Design review of the part built by this model. Coordinates are the model's own, in mm. Face numbers are marked on the shaded views. Coordinates: 2 decimals unless noted, no trailing zeros. Loops run counter-clockwise (first coordinate to the right, second up) from the corner with the lowest first, then second, coordinate; pieces in that order, holes last. Notation, with made-up numbers: (22.25, 16) -> (28.25, 16) arc R33 ccw to (28.25, 45) -> close; hole circle Ø5 at (44.5, 47.5). An arc over 180 degrees is marked (long way). Answer as a JSON object with one key per item and string values.
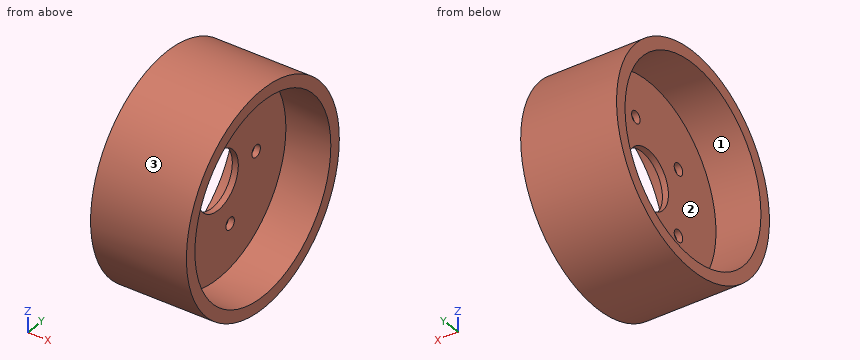
```python
from build123d import *

# Parameters (mm, degrees)
SKETCH1_W                  = 6.35
SKETCH1_H                  = 101.6
SKETCH2_R                  = 30.48
CUT_EXTRUDE2_DEPTH         = 171.417958634
F_1_2_0_5_DIAMETER_HOLE2_D = 12.7


with BuildPart() as part:
    # Sketch1 → Revolve1 (revolve)
    with BuildSketch(Plane.XY):
        with Locations((3.175, 50.8)):
            Rectangle(SKETCH1_W, SKETCH1_H)
        Polygon((-47.625, 101.6), (0, 101.6), (6.35, 101.6), (53.975, 101.6), (53.975, 114.3), (-47.625, 114.3), align=None)
    revolve(axis=Axis((6.35, 0, 0), (-1, 0, 0)))

    # Sketch2 → Cut-Extrude2 (cut, through all)
    with BuildSketch(Plane(origin=(6.35, 0, 0), x_dir=(0, 0, -1), z_dir=(1, 0, 0))):
        with Locations(Location((0, 0, 0), (0, 0, 90))):
            Circle(SKETCH2_R)
    extrude(amount=-CUT_EXTRUDE2_DEPTH, mode=Mode.SUBTRACT)

    # 1/2 (0.5) Diameter Hole2 (through all)
    with Locations(Plane(origin=(6.35, 0, 0), x_dir=(0, 0, -1), z_dir=(1, 0, 0))):
        with Locations((-54.155626078, 18.25625), (0, 57.15), (54.155626078, 18.25625), (34.599427772, -45.486284722), (-34.599427772, -45.486284722)):
            Hole(F_1_2_0_5_DIAMETER_HOLE2_D / 2)


solid = part.part
```
1) Clearance check with flat-ended pins moving along their axes: pin 1 Ø10 at (x, z) = (37, 73) entering from -Y; pin 2 Ø3 at (x, y) = (-10, 56.5) entering from -Z; pin 3 Ø8 at (x, z) = (25.5, -55.5) entering from -Y. State where each tip first meets the part, or that it passes through.
Completed:
{"pin 1": "y = -91.87", "pin 2": "z = -100.2", "pin 3": "y = -102.04"}
2) The part is to be moulded in two halves that separate along Z. For the marked faces 1, 2 and 3, say which applies: pulls with the +Z half, pulls with the -Z half, needs draft (parallel to the pull), parting line crosses it, or undercut.
Completed:
{"face 1": "undercut", "face 2": "undercut", "face 3": "parting line crosses it"}
3) Add section A-A, the plane z = 0. Give the boundary of the cut face in (x, y) (3 decimals), and give its area (3 significant figures).
Completed:
{"outline": "(-47.625, -114.3) -> (53.975, -114.3) -> (53.975, -101.6) -> (6.35, -101.6) -> (6.35, -30.48) -> (0, -30.48) -> (0, -101.6) -> (-47.625, -101.6) -> close; (-47.625, 101.6) -> (0, 101.6) -> (0, 63.5) -> (6.35, 63.5) -> (6.35, 101.6) -> (53.975, 101.6) -> (53.975, 114.3) -> (-47.625, 114.3) -> close; (0, 30.48) -> (6.35, 30.48) -> (6.35, 50.8) -> (0, 50.8) -> close", "area": "3,400 mm²"}
4) Add section D-D, the plane y = 38.5. Give the boundary of the cut face in (x, z) (3 decimals).
Completed:
{"outline": "(-47.625, -107.621) -> (53.975, -107.621) -> (53.975, -94.023) -> (6.35, -94.023) -> (6.35, 94.023) -> (53.975, 94.023) -> (53.975, 107.621) -> (-47.625, 107.621) -> (-47.625, 94.023) -> (0, 94.023) -> (0, -94.023) -> (-47.625, -94.023) -> close"}
5) Add section B-B, the plane y = 0. Give the boundary of the cut face in (x, z) (3 decimals), and give its area (3 significant figures).
Completed:
{"outline": "(-47.625, -114.3) -> (53.975, -114.3) -> (53.975, -101.6) -> (6.35, -101.6) -> (6.35, -30.48) -> (0, -30.48) -> (0, -101.6) -> (-47.625, -101.6) -> close; (-47.625, 101.6) -> (0, 101.6) -> (0, 30.48) -> (6.35, 30.48) -> (6.35, 101.6) -> (53.975, 101.6) -> (53.975, 114.3) -> (-47.625, 114.3) -> close", "area": "3,480 mm²"}
6) Add section C-C, the plane x = 34. Give the boundary of the cut face in (y, z), and give its area (3 significant figures).
Completed:
{"outline": "circle Ø228.6 at (0, 0); hole circle Ø203.2 at (0, 0)", "area": "8,610 mm²"}
7) Wall thickness on probe 1 along Z at (x, y) = (-19, 0); probe 2 along Z at (x, y) = (38.5, 68); probe 3 along Y at (x, z) = (-13.5, -85): over which ranges is each line inside the solid? List them lowest first.
Completed:
{"probe 1": "-114.3 to -101.6, 101.6 to 114.3", "probe 2": "-91.87 to -75.49, 75.49 to 91.87", "probe 3": "-76.42 to -55.66, 55.66 to 76.42"}
